from build123d import *

# Parameters (mm, degrees)
SKETCH007_R     = 2.125
PAD002_DEPTH    = 8
POCKET005_DEPTH = 73.701
CHAMFER003_SIZE = 1


with BuildPart() as part:
    # Sketch007 → Pad002 (new body)
    with BuildSketch(Plane.XY):
        with BuildLine():
            ThreePointArc((0, -14.35), (14.35, 0), (0, 14.35))
            Line((0, 14.35), (-20, 14.35))
            ThreePointArc((-21.414214, 14.935786), (-20.765367, 14.502241), (-20, 14.35))
            Line((-21.414214, 14.935786), (-26.730188, 20.251761))
            ThreePointArc((-27.315974, 21.665974), (-27.163734, 20.900608), (-26.730188, 20.251761))
            Line((-27.315974, 21.665974), (-27.315974, 57.22868))
            Line((-27.315974, 57.22868), (-29.437295, 59.35))
            Line((-56.015974, 59.35), (-29.437295, 59.35))
            Line((-56.015974, 21.665974), (-56.015974, 59.35))
            ThreePointArc((-56.015974, 21.665974), (-54.923646, 16.174467), (-51.812957, 11.518992))
            Line((-51.812957, 11.518992), (-30.146982, -10.146982))
            ThreePointArc((-30.146982, -10.146982), (-25.491507, -13.257671), (-20, -14.35))
            Line((-20, -14.35), (0, -14.35))
        make_face()
        with Locations((-35.690974, 50.975)):
            Circle(SKETCH007_R, mode=Mode.SUBTRACT)
        with Locations((-35.690974, 40.475)):
            Circle(SKETCH007_R, mode=Mode.SUBTRACT)
        with Locations((-35.690974, 29.975)):
            Circle(SKETCH007_R, mode=Mode.SUBTRACT)
        with BuildLine():
            ThreePointArc((0, 6.25), (1.55, 7.8), (0, 9.35))
            Line((-20, 9.35), (0, 9.35))
            ThreePointArc((-20, 9.35), (-21.55, 7.8), (-20, 6.25))
            Line((-20, 6.25), (0, 6.25))
        make_face(mode=Mode.SUBTRACT)
        with BuildLine():
            ThreePointArc((-20, -6.25), (-21.55, -7.8), (-20, -9.35))
            Line((-20, -9.35), (0, -9.35))
            ThreePointArc((0, -9.35), (1.55, -7.8), (0, -6.25))
            Line((-20, -6.25), (0, -6.25))
        make_face(mode=Mode.SUBTRACT)
        with BuildLine():
            ThreePointArc((7.8, -1.55), (9.35, 0), (7.8, 1.55))
            Line((5.015974, 1.55), (7.8, 1.55))
            ThreePointArc((5.015974, 1.55), (3.116488, 4.224926), (0, 5.25))
            Line((-20, 5.25), (0, 5.25))
            ThreePointArc((-20, 5.25), (-23.116488, 4.224926), (-25.015974, 1.55))
            Line((-27.8, 1.55), (-25.015974, 1.55))
            ThreePointArc((-27.8, 1.55), (-29.35, 0), (-27.8, -1.55))
            Line((-27.8, -1.55), (-25.015974, -1.55))
            ThreePointArc((-25.015974, -1.55), (-23.116488, -4.224926), (-20, -5.25))
            Line((-20, -5.25), (0, -5.25))
            ThreePointArc((0, -5.25), (3.116488, -4.224926), (5.015974, -1.55))
            Line((7.8, -1.55), (5.015974, -1.55))
        make_face(mode=Mode.SUBTRACT)
    extrude(amount=PAD002_DEPTH)

    # Sketch008 (on Face12 of Pad002) → Pocket005 (cut, through all)
    with BuildSketch(Plane(origin=(0, 59.35, 0), x_dir=(-1, 0, 0), z_dir=(0, 1, 0))):
        with BuildLine():
            Line((56.015974, 7), (47.765974, 7))
            ThreePointArc((44.015974, 7), (45.890974, 5.125), (47.765974, 7))
            Line((44.015974, 8), (44.015974, 7))
            Line((44.015974, 8), (56.015974, 8))
            Line((56.015974, 8), (56.015974, 7))
        make_face()
    extrude(amount=-POCKET005_DEPTH, mode=Mode.SUBTRACT)

    # Chamfer003
    chamfer003_edges = [part.edges().sort_by_distance(p)[0] for p in [
        (-42.726635, 59.35, 0),
        (-56.015974, 40.507987, 0),
        (-54.923646, 16.174467, 0),
        (-40.97997, 0.686005, 0),
        (-25.491507, -13.257671, 0),
        (-10, -14.35, 0),
        (14.35, 0, 0),
        (-10, 14.35, 0),
        (-20.765367, 14.502241, 0),
        (-24.072201, 17.593774, 0),
        (-27.163734, 20.900608, 0),
        (-27.315974, 39.447327, 0),
        (-28.376635, 58.28934, 0),
    ]]
    chamfer(chamfer003_edges, length=CHAMFER003_SIZE)


with BuildPart() as part_1:
    # Body002 placement: moved
    add(part.part.moved(Location((11, 3.5, 0))))


solid = part_1.part
For this review, take the finished solid that the model builds, in its own axes (mm). A direction names the side the tool comes from. Give positions to 0.01 mm unless a question says otherwise; leave off trailing zeros. Loops run counter-clockwise (first coordinate to the right, second up) from the corner with the lowest first, then second, coordinate; pieces in that order, holes last. Notation, with made-up numbers: M 67,-37.75 L 91,-37.75 A14 cw 91,-24.75 Z; hole C 63.25,43.5 d5. An arc over 180 degrees is marked long. Put each result on its own line as item: value. Start each with the question number.
(1) Machinability: for faces 4 (the flat face through (1, 17.85, 4)), 5 (the flat face through (1, -5.85, 4)), 6 (the cylindrical face through (25.347, 3.184, 4.451)), which of the approach directions +Z, -Z, +X, -X, +Y, -Y give a long, thin tool a straight path to every point of the face, cutting with its end or side? Answer none if there is none.
(2) Wall thickness on L1, parallel to Y at x = 8.5, z = 4.75; L2, parallel to X at y = -0.5, z = 1.5: over which ranges is each line inside the solid? List them lowest first.
(3) The part is to be moulded in two halves that separate along Y. For faces 1 (the conical face through (24.52, 3.797, 0.174)), 2 (the flat face through (-13.035, 21.057, 4.451)), 3 (the cylindrical face through (-18.35, 3.53, 3.94)), say which applies: +Y half, -Y half, draft (parallel to the pull), parting line (faces both ways), or undercut.
(4) Add section B-B, the plane y = 3.5. Write out the cut boundary in (x, z), then the cut area to 3 significant figures.
(5) Add section A-A, the plane y = 26. Write out the cut boundary in (x, z) (3 decimals).
(6) Add section C-C, the plane z = 3.5. Give the number of separate pieces and of enclosed holes in the cut face, then the cut area to 3 significant figures.
(7) For pin 1 (0.5 mm diameter, centred on y = 27, z = 7.5, fed in from -X); pin 2 (3 mm diameter, centred on x = -15, z = 2.5, fed in from -Y); pin 3 (4 mm diameter, centred on x = -42.5, y = 46.5, fed in from +Z); pin 4 (4 mm diameter, centred on x = -24.69, y = 54.48, fed in from +Z), all flat-tipped, find the tip position at first contact; note any pin that passes through.
Result:
1. face 4: +Z, -Z, +X, +Y
1. face 5: +Z, -Z
1. face 6: +Z, -Z, +X
2. L1: y = -10.85 to -5.85, -2.75 to -1.75, 8.75 to 9.75, 12.85 to 17.85
2. L2: x = -25.29 to -12.4, 14.4 to 24.78
3. face 1: parting line
3. face 2: +Y half
3. face 3: undercut
4. outline: M -29.29,1 L -27.88,0 L -18.35,0 L -18.35,8 L -29.29,8 Z; M 20.35,0 L 24.35,0 L 25.35,1 L 25.35,8 L 20.35,8 Z
4. area: 126 mm^2
5. outline: M -45.016,1 L -44.016,0 L -17.316,0 L -16.316,1 L -16.316,8 L -33.016,8 L -33.016,7 A1.875 cw -36.766,7 L -45.016,7 Z
6. separate pieces: 1
6. enclosed holes: 6
6. area: 2,280 mm^2
7. pin 1: stops at x = -33.02
7. pin 2: stops at y = -10.13
7. pin 3: stops at z = 7
7. pin 4: passes through
